The model under review builds one solid part; all positions refer to its coordinate system, in mm. A direction names the side the tool comes from. Give positions to 0.01 mm unless a question says otherwise; leave off trailing zeros. Order: outer loops, then holes, each group sorted by start corner. A loop starts at its lowest first (then second) coordinate and runs counter-clockwise, first axis right, second up. Notation, with made-up numbers: (51, 27) -> (99, 27) arc R20 ccw to (99, 56) -> close; hole circle Ø1 at (59.25, 22). An arc over 180 degrees is marked (long way). Use one line per item in the form item = value.
```python
from build123d import *

# Parameters (mm, degrees)
F0_W      = 120
F0_H      = 120
F0_R      = 1.5
F1_DEPTH  = 1.75
F2_R      = 2.75
F2_R_2    = 1.5
F3_DEPTH  = 15
F4_R      = 2
F4_R_2    = 1.5
F5_DEPTH  = 1
F4_R_3    = 1.75
F6_DEPTH  = 4.35
F7_W      = 74.1
F7_H      = 64.1
F8_DEPTH  = 1.75
F9_R      = 2
F10_DEPTH = 1
F9_W      = 30
F9_H      = 30
F11_DEPTH = 7
F12_R     = 10.5
F12_W     = 6.5
F12_H     = 4
F13_DEPTH = 1
F12_W_2   = 1.5
F12_H_2   = 1.5
F14_DEPTH = 0.3
F15_DEPTH = 0.5


with BuildPart() as f1:
    # F0 (on Top) → F1 (new body)
    with BuildSketch(Plane.XY):
        Rectangle(F0_W, F0_H)
        with Locations((-56.5, -56.5)):
            Circle(F0_R, mode=Mode.SUBTRACT)
        with Locations((56.5, -56.5)):
            Circle(F0_R, mode=Mode.SUBTRACT)
        with Locations((-56.5, 56.5)):
            Circle(F0_R, mode=Mode.SUBTRACT)
        with Locations((56.5, 56.5)):
            Circle(F0_R, mode=Mode.SUBTRACT)
    extrude(amount=F1_DEPTH)

    # F2 (on face) → F3 (join)
    with BuildSketch(Plane(origin=(0, 0, 0), x_dir=(1, 0, 0), z_dir=(0, 0, -1))):
        with Locations((56.5, -56.5)):
            Circle(F2_R)
        with Locations((56.5, -56.5)):
            Circle(F2_R_2, mode=Mode.SUBTRACT)
        with Locations((-56.5, -56.5)):
            Circle(F2_R)
        with Locations((-56.5, -56.5)):
            Circle(F2_R_2, mode=Mode.SUBTRACT)
        with Locations((-56.5, 56.5)):
            Circle(F2_R)
        with Locations((-56.5, 56.5)):
            Circle(F2_R_2, mode=Mode.SUBTRACT)
        with Locations((56.5, 56.5)):
            Circle(F2_R)
        with Locations((56.5, 56.5)):
            Circle(F2_R_2, mode=Mode.SUBTRACT)
        with Locations((-56.5, 56.5)):
            Circle(F2_R_2)
        with Locations((56.5, 56.5)):
            Circle(F2_R_2)
        with Locations((-56.5, -56.5)):
            Circle(F2_R_2)
        with Locations((56.5, -56.5)):
            Circle(F2_R_2)
    extrude(amount=F3_DEPTH)

    # F4 (on face) → F5 (join)
    with BuildSketch(Plane.XY.offset(1.75)):
        with Locations((-56.5, 56.5)):
            Circle(F4_R)
        with Locations((-56.5, 56.5)):
            Circle(F4_R_2, mode=Mode.SUBTRACT)
        with Locations((-56.5, 56.5)):
            Circle(F4_R_2)
        with Locations((56.5, 56.5)):
            Circle(F4_R)
        with Locations((56.5, 56.5)):
            Circle(F4_R_2, mode=Mode.SUBTRACT)
        with Locations((56.5, 56.5)):
            Circle(F4_R_2)
        with Locations((56.5, -56.5)):
            Circle(F4_R)
        with Locations((56.5, -56.5)):
            Circle(F4_R_2, mode=Mode.SUBTRACT)
        with Locations((56.5, -56.5)):
            Circle(F4_R_2)
        with Locations((-56.5, -56.5)):
            Circle(F4_R)
        with Locations((-56.5, -56.5)):
            Circle(F4_R_2, mode=Mode.SUBTRACT)
        with Locations((-56.5, -56.5)):
            Circle(F4_R_2)
    extrude(amount=F5_DEPTH)

    # F4 (on face) → F6 (join)
    with BuildSketch(Plane.XY.offset(1.75)):
        with Locations((-33.55, -28.55)):
            Circle(F4_R_3)
        with Locations((33.55, -28.55)):
            Circle(F4_R_3)
        with Locations((33.55, 28.55)):
            Circle(F4_R_3)
        with Locations((-33.55, 28.55)):
            Circle(F4_R_3)
    extrude(amount=F6_DEPTH)

    # F7 (on face) → F8 (join)
    with BuildSketch(Plane.XY.offset(6.1)):
        Rectangle(F7_W, F7_H)
    extrude(amount=F8_DEPTH)

    # F9 (on face) → F10 (join)
    with BuildSketch(Plane.XY.offset(7.85)):
        with Locations((33.55, 28.55)):
            Circle(F9_R)
        with Locations((-33.55, 28.55)):
            Circle(F9_R)
        with Locations((33.55, -28.55)):
            Circle(F9_R)
        with Locations((-33.55, -28.55)):
            Circle(F9_R)
    extrude(amount=F10_DEPTH)

    # F9 (on face) → F11 (join)
    with BuildSketch(Plane.XY.offset(7.85)):
        Rectangle(F9_W, F9_H)
    extrude(amount=F11_DEPTH)

    # F12 (on face) → F13 (cut)
    with BuildSketch(Plane.XY.offset(14.85)):
        Circle(F12_R)
        Rectangle(F12_W, F12_H, mode=Mode.SUBTRACT)
    extrude(amount=-F13_DEPTH, mode=Mode.SUBTRACT)

    # F12 (on face) → F14 (cut)
    with BuildSketch(Plane.XY.offset(14.85)):
        Rectangle(F12_W_2, F12_H_2)
    extrude(amount=-F14_DEPTH, mode=Mode.SUBTRACT)

    # F12 (on face) → F15 (cut)
    with BuildSketch(Plane.XY.offset(14.85)):
        Rectangle(F12_W, F12_H)
        Rectangle(F12_W_2, F12_H_2, mode=Mode.SUBTRACT)
    extrude(amount=-F15_DEPTH, mode=Mode.SUBTRACT)


solid = f1.part
```
1. Add section A-A on y = 25. Give the boundary of the cut face in (x, z).
Values:
outline = (-60, 0) -> (60, 0) -> (60, 1.75) -> (-60, 1.75) -> close; (-37.05, 6.1) -> (37.05, 6.1) -> (37.05, 7.85) -> (-37.05, 7.85) -> close
2. Add section C-C on y = -28.55. Give the boundary of the cut face in (x, z), then the cut area to 3 significant figures.
Values:
outline = (-60, 0) -> (60, 0) -> (60, 1.75) -> (35.3, 1.75) -> (35.3, 6.1) -> (37.05, 6.1) -> (37.05, 7.85) -> (35.55, 7.85) -> (35.55, 8.85) -> (31.55, 8.85) -> (31.55, 7.85) -> (-31.55, 7.85) -> (-31.55, 8.85) -> (-35.55, 8.85) -> (-35.55, 7.85) -> (-37.05, 7.85) -> (-37.05, 6.1) -> (-35.3, 6.1) -> (-35.3, 1.75) -> (-60, 1.75) -> close; hole (-31.8, 1.75) -> (31.8, 1.75) -> (31.8, 6.1) -> (-31.8, 6.1) -> close
area = 378 mm^2
3. Add section D-D on x = -56.5. Give the boundary of the cut face in (y, z).
Values:
outline = (-60, 0) -> (-59.25, 0) -> (-59.25, -15) -> (-53.75, -15) -> (-53.75, 0) -> (53.75, 0) -> (53.75, -15) -> (59.25, -15) -> (59.25, 0) -> (60, 0) -> (60, 1.75) -> (58.5, 1.75) -> (58.5, 2.75) -> (54.5, 2.75) -> (54.5, 1.75) -> (-54.5, 1.75) -> (-54.5, 2.75) -> (-58.5, 2.75) -> (-58.5, 1.75) -> (-60, 1.75) -> close; hole (-58, 0) -> (-55, 0) -> (-55, 1.75) -> (-58, 1.75) -> close; hole (55, 0) -> (58, 0) -> (58, 1.75) -> (55, 1.75) -> close
4. Add section B-B on x = -28.5. Give the boundary of the cut face in (y, z), then the cut area to 3 significant figures.
Values:
outline = (-60, 0) -> (60, 0) -> (60, 1.75) -> (-60, 1.75) -> close; (-32.05, 6.1) -> (32.05, 6.1) -> (32.05, 7.85) -> (-32.05, 7.85) -> close
area = 322 mm^2
5. For L1, parallel to Y at x = 56.5, z = 0.95; L2, parallel to Z at x = 23, y = 4.5; L3, parallel to Z at x = 5, y = -7, list the stretches that pass through material, from the lowest coordinate up.
Values:
L1 = -60 to -58, -55 to 55, 58 to 60
L2 = 0 to 1.75, 6.1 to 7.85
L3 = 0 to 1.75, 6.1 to 13.85
6. The part is to be moulded in two halves that separate along X. For faces 1 (the face through (-57, 57, 2.75)), 2 (the face through (56, 56, 0)), 3 (the face through (-15, 0, 11)), say which applies: +X half, -X half, draft (parallel to the pull), parting line (faces both ways), or undercut.
Values:
face_1 = draft
face_2 = undercut
face_3 = -X half
7. For pin 1 Ø12 at (x, y) = (-48, -40) entering from +Z; pin 2 Ø1.8 at (x, y) = (56.5, 56.5) entering from +Z; pin 3 Ø0.9 at (x, z) = (7.5, 7.5) entering from +Y; pin 4 Ø4 at (x, y) = (-15.5, -15.5) entering from +Z, all flat-tipped, find the tip position at first contact; note any pin that passes through.
Values:
pin_1 = 1.75
pin_2 = 2.75
pin_3 = 32.05
pin_4 = 14.85
8. Tool access review of faces 4 (the face through (-57, -57, -15)), 5 (the face through (0, -15, 11)), 6 (the face through (56.24, -54.517, 2.243)), 7 (the face through (-57, -56, 2.75)), 8 (the face through (-57, 57, 1.75)): name each direction out of +Z, -Z, +X, -X, +Y, -Y from which nothing blocks a thin tool from reaching the whole face with its end or side.
Values:
face_4 = -Z, +X, -X, +Y, -Y
face_5 = +Z, +X, -X, -Y
face_6 = +Z
face_7 = +Z, +X, -X, +Y, -Y
face_8 = none
